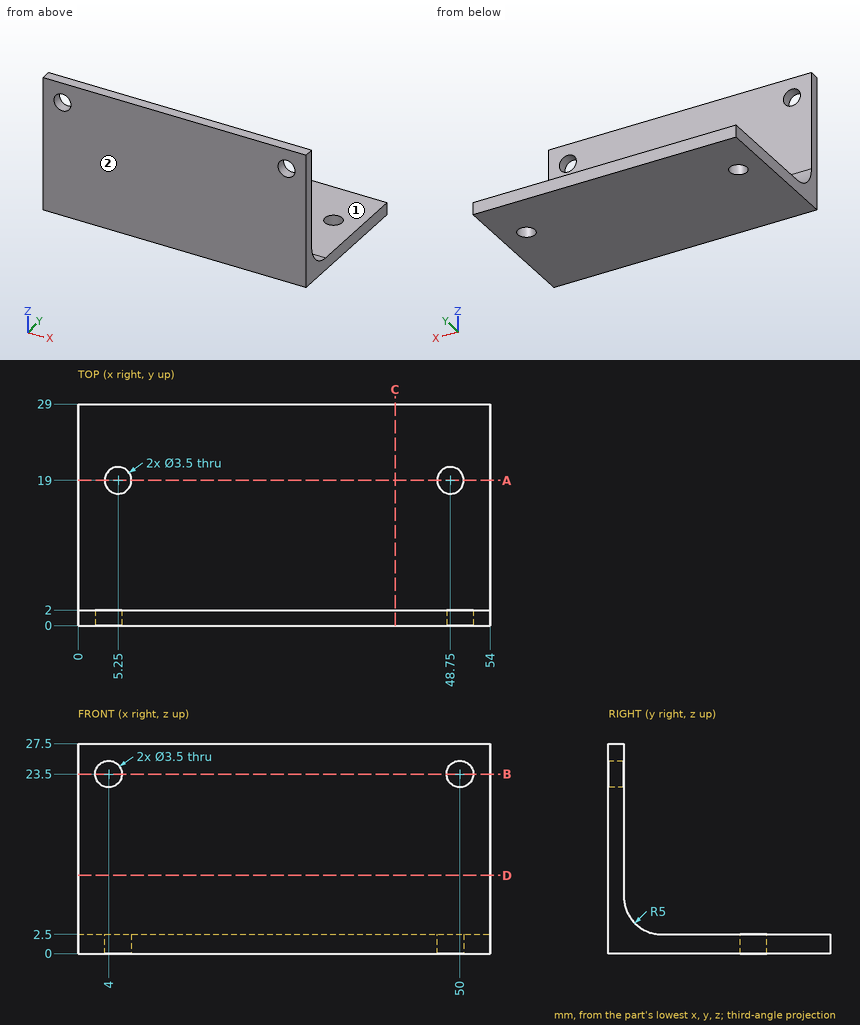
Job drawing, mm, ordinate dimensions from the low corner. One solid piece. A direction names the side the tool comes from. Give positions to 0.01 mm unless a question says otherwise; leave off trailing zeros. Loops run counter-clockwise (first coordinate to the right, second up) from the corner with the lowest first, then second, coordinate; pieces in that order, holes last. Notation, with made-up numbers: M 71.25,-19.75 L 81.25,-19.75 A21 cw 81.25,-13.75 Z; hole C -15,57 d10. An arc over 180 degrees is marked long. Put each result on its own line as item: value. Start each with the question number.
1) Saw through at C-C (x = 41.5). List the corners of the cut face in (y, z).
2) Saw through at A-A (y = 19). List the corners of the cut face in (x, z).
3) 3-axis set-ups, long thin cutter, end or side, ignore diameter. For the marked faces 1 and 2: which of +Z, -Z, +X, -X, +Y, -Y reach the whole face in a straight line?
4) Saw through at B-B (z = 23.5). List the corners of the cut face in (x, y), then the cut area to 3 significant figures.
5) Probe probe 1 along Y at (x, z) = (5.25, 1.7); probe 2 along X at (y, z) = (0.8, 23.5); probe 3 along Y at (x, z) = (15, 24). List the from-to ranges inside material, lowest first.
6) Saw through at D-D (z = 10.25). List the corners of the cut face in (x, y), then the cut area to 3 significant figures.
7) Flat gauge pins, fed straight in: pin 1 (6 mm diameter, centred on x = 40.5, z = 18, fed in from -Y); pin 2 (16 mm diameter, centred on x = 20.5, z = 17.5, fed in from +Y); pin 3 (3 mm diameter, centred on x = 4, z = 23.5, fed in from -Y); pin 4 (4 mm diameter, centred on x = 5.25, y = 19, fed in from +Z). Where does each tip first touch, or does it go through?
Numbers:
1. outline: M 0,0 L 29,0 L 29,2.5 L 7,2.5 A5 cw 2,7.5 L 2,27.5 L 0,27.5 Z
2. outline: M 0,0 L 3.5,0 L 3.5,2.5 L 0,2.5 Z; M 7,0 L 47,0 L 47,2.5 L 7,2.5 Z; M 50.5,0 L 54,0 L 54,2.5 L 50.5,2.5 Z
3. face 1: +Z, +X, -X, +Y
3. face 2: +Z, -Z, +X, -X, -Y
4. outline: M 0,0 L 2.25,0 L 2.25,2 L 0,2 Z; M 5.75,0 L 48.25,0 L 48.25,2 L 5.75,2 Z; M 51.75,0 L 54,0 L 54,2 L 51.75,2 Z
4. area: 94.0 mm^2
5. probe 1: 0 to 17.25, 20.75 to 29
5. probe 2: 0 to 2.25, 5.75 to 48.25, 51.75 to 54
5. probe 3: 0 to 2
6. outline: M 0,0 L 54,0 L 54,2 L 0,2 Z
6. area: 108 mm^2
7. pin 1: y = 0
7. pin 2: y = 2
7. pin 3: through
7. pin 4: z = 2.5
